Model file for the job. Use its own axes, mm. Face numbers are marked on the shaded views. A direction names the side the tool comes from. Coordinates: 2 decimals unless noted, no trailing zeros. Order: outer loops, then holes, each group sorted by start corner. A loop starts at its lowest first (then second) coordinate and runs counter-clockwise, first axis right, second up. Notation, with made-up numbers: (84, -35) -> (90, -35) arc R21 ccw to (90, -12) -> close; hole circle Ø5 at (61.5, -14.5). An arc over 180 degrees is marked (long way). Write item = value, one per line. Start each with the question number.
Q1. Cut at B-B, the plane y = -43. List the corners of the cut face in (x, z).
Q2. Flat gauge pins, fed straight in: pin 1 (5 mm diameter, centred on x = 0.5, y = -53, fed in from +Z); pin 2 (5 mm diameter, centred on y = -55.5, z = -4, fed in from +X); pin 3 (5 mm diameter, centred on x = 10.5, z = 2, fed in from +Y). Where does each tip first touch, or does it go through?
Q3. 3-axis set-ups, long thin cutter, end or side, ignore diameter. For the marked faces 1 and 2: which of +Z, -Z, +X, -X, +Y, -Y reach the whole face in a straight line?
Q4. Mould opens along Y. For the marked faces 3, 4, 5 and 6 say: +Y half, -Y half, draft (parallel to the pull), parting line (faces both ways), or undercut.
Q5. Wall check: line 1 (Y direction, x = -21, z = -3.5); line 2 (X direction, y = -72.4, z = 0); line 3 (X direction, y = -1.95, z = 0). Give the ranges that are in metal, low to high. Write a range as from..to.
Q6. Cut at A-A, the plane x = 20. List the corners of the cut face in (y, z), plus the area to 3 significant figures.
from build123d import *

# Parameters (mm, degrees)
BASE_FLANGE1_START  = -5
BASE_FLANGE1_DEPTH  = 10
SKETCH7_R           = 2.5
CUT_EXTRUDE2_DEPTH  = 10
BOSS_EXTRUDE1_START = 1
BOSS_EXTRUDE1_DEPTH = 2
BOSS_EXTRUDE1_DRAFT = -15
BOSS_EXTRUDE2_DEPTH = 54.4
BOSS_EXTRUDE3_START = 4
SKETCH10_W          = 50
SKETCH10_H          = 12.5
SKETCH10_R          = 2.5
BOSS_EXTRUDE3_DEPTH = 4


# Read off the part's stored shape, not the designer's step: Base-Flange1
with BuildPart() as part:
    # Base-Flange1 outline → Base-Flange1 (new body)
    with BuildSketch(Plane.XY.offset(BASE_FLANGE1_START)):
        with BuildLine():
            Line((-16.314153364, 0), (-25, 0))
            Line((-25, 0), (-25, -3))
            Line((-25, -3), (-16.314153364, -3))
            ThreePointArc((-16.314153364, -3), (-15.855108879, -3.160529066), (-15.596145802, -3.57214727))
            ThreePointArc((-15.596145802, -3.57214727), (0, -16), (15.596145802, -3.57214727))
            ThreePointArc((15.596145802, -3.57214727), (15.855108879, -3.160529066), (16.314153364, -3))
            Line((16.314153364, -3), (25, -3))
            Line((25, -3), (25, 0))
            Line((25, 0), (16.314153364, 0))
            ThreePointArc((16.314153364, 0), (13.985527754, -0.814326513), (12.671868464, -2.902369657))
            ThreePointArc((12.671868464, -2.902369657), (0, -13), (-12.671868464, -2.902369657))
            ThreePointArc((-12.671868464, -2.902369657), (-13.985527754, -0.814326513), (-16.314153364, 0))
        make_face()
    extrude(amount=BASE_FLANGE1_DEPTH)

    # Sketch7 → Cut-Extrude2 (cut)
    with BuildSketch(Plane.XZ.offset(3)):
        with Locations(Location((-20, 0, 0), (0, 0, 270))):
            Circle(SKETCH7_R)
    cut_extrude2 = extrude(amount=-CUT_EXTRUDE2_DEPTH, mode=Mode.SUBTRACT)

    # Mirror1: Cut-Extrude2 across plane
    add(cut_extrude2.mirror(Plane(origin=(0, 0, 0), x_dir=(0, 0, 1), z_dir=(1, 0, 0))), mode=Mode.SUBTRACT)


with BuildPart() as boss_extrude1_tool:
    # Sketch8 → Boss-Extrude1 (with draft: the straight prism first)
    with BuildSketch(Plane(origin=(0, -16, 0), x_dir=(-1, 0, 0), z_dir=(0, -1, 0)).offset(BOSS_EXTRUDE1_START)):
        Polygon((-2.25, -3.897114317), (2.25, -3.897114317), (4.5, 0), (2.25, 3.897114317), (-2.25, 3.897114317), (-4.5, 0), align=None)
    extrude(amount=-BOSS_EXTRUDE1_DEPTH)
    # Boss-Extrude1: the draft: its side faces are tilted about the plane it starts from
    boss_extrude1_sides = [boss_extrude1_tool.faces().sort_by_distance(p)[0] for p in [
        (0, -16, 3.897114317),
        (-3.375, -16, 1.948557159),
        (-3.375, -16, -1.948557159),
        (0, -16, -3.897114317),
        (3.375, -16, -1.948557159),
        (3.375, -16, 1.948557159),
    ]]
    draft(boss_extrude1_sides, Plane(origin=(0, -16, 0), x_dir=(-1, 0, 0), z_dir=(0, -1, 0)).offset(BOSS_EXTRUDE1_START), BOSS_EXTRUDE1_DRAFT)


with BuildPart() as part_1:
    add(part.part)

    # Boss-Extrude1: add boss_extrude1_tool
    add(boss_extrude1_tool.part)

    # Sketch9 → Boss-Extrude2 (add)
    with BuildSketch(Plane.XZ.offset(17)):
        Polygon((4.5, 0), (2.25, 3.897114317), (-2.25, 3.897114317), (-4.5, 0), (-2.25, -3.897114317), (2.25, -3.897114317), align=None)
    extrude(amount=BOSS_EXTRUDE2_DEPTH)

    # Sketch10 → Boss-Extrude3 (add)
    with BuildSketch(Plane.XZ.offset(71.4).offset(BOSS_EXTRUDE3_START)):
        Rectangle(SKETCH10_W, SKETCH10_H)
        with Locations(Location((-20, 0, 0), (0, 0, 270))):
            Circle(SKETCH10_R, mode=Mode.SUBTRACT)
        with Locations(Location((20, 0, 0), (0, 0, 270))):
            Circle(SKETCH10_R, mode=Mode.SUBTRACT)
    extrude(amount=-BOSS_EXTRUDE3_DEPTH)


solid = part_1.part
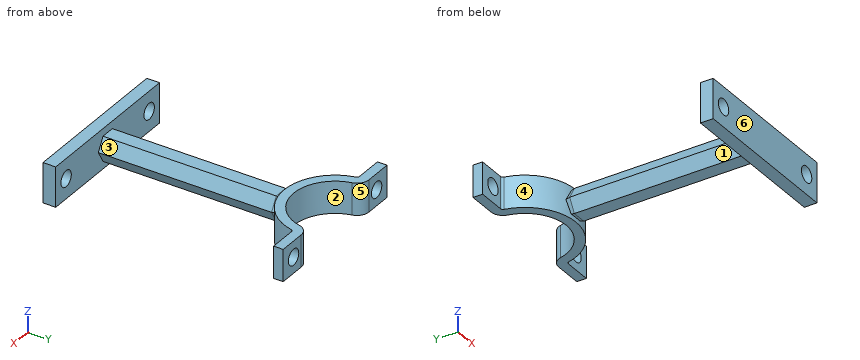
Here are the results:
q1.outline = (-4.5, 0) -> (-2.25, -3.9) -> (2.25, -3.9) -> (4.5, 0) -> (2.25, 3.9) -> (-2.25, 3.9) -> close
q2.pin_1 = 3.9
q2.pin_2 = 3.63
q2.pin_3 = -2.01
q3.face_1 = -Z, -X
q3.face_2 = +Z, -Z, +Y
q4.face_3 = undercut
q4.face_4 = undercut
q4.face_5 = +Y half
q4.face_6 = -Y half
q5.line_1 = -75.4..-71.4, -3..0
q5.line_2 = -25..-22.5, -17.5..17.5, 22.5..25
q5.line_3 = -25..-22.5, -17.5..-13.03, 13.03..17.5, 22.5..25
q6.outline = (-75.4, -6.25) -> (-71.4, -6.25) -> (-71.4, -2.5) -> (-75.4, -2.5) -> close; (-75.4, 2.5) -> (-71.4, 2.5) -> (-71.4, 6.25) -> (-75.4, 6.25) -> close; (-3, -5) -> (0, -5) -> (0, -2.5) -> (-3, -2.5) -> close; (-3, 2.5) -> (0, 2.5) -> (0, 5) -> (-3, 5) -> close
q6.area = 45.0 mm²
